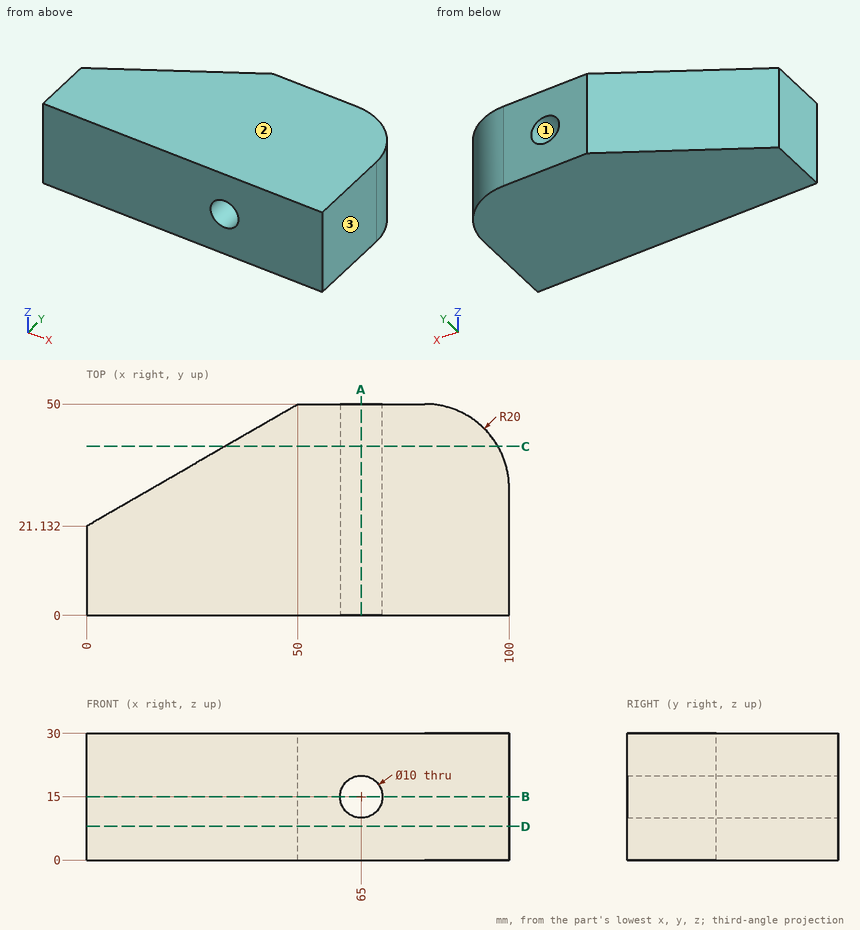
Geometry: see drawing. Coordinates: mm, zero at the bounding-box minimum. Coordinates: 2 decimals unless noted, no trailing zeros. Order: outer loops, then holes, each group sorted by start corner. A loop starts at its lowest first (then second) coordinate and runs counter-clockwise, first axis right, second up. Notation, with made-up numbers: M 67,61.5 L 94,61.5 A14 ccw 94,83.5 Z; hole C 12,51.5 d1. An arc over 180 degrees is marked long. Answer in a Markdown table with one row per item. Add a question column.
Q1. Section query B-B on z = 15. Return the cut outline in (x, y).
Q2. Line query: L1, parallel to Z at x = 65, y = 20; L2, parallel to X at y = 40, z = 16 (1 decimal); L3, parallel to Z at x = 66.5, y = 8. Output: solid intervals per line, ascending.
Q3. Mould query, pull axis Z, two halves, no side actions, for the marked faces 1, 2 and 3. Classes: released by +Z, released by -Z, zero draft, split by the parting line, or undercut.
Q4. Section query D-D on z = 8. Return the cut outline in (x, y), and give its area (3 significant figures).
Q5. Contact query for a flat-ended pin moving along its axis: P1, Ø8, axis at y = 44.5, z = 22, coming from the +X side. Output: stop coordinate, or through.
Q6. Section query C-C on y = 40. Return the cut outline in (x, z).
Q7. Section query A-A on x = 65. Return the cut outline in (y, z), and give its area (3 significant figures).
Completed:
| question | item | result |
|---|---|---|
| 1 | outline | M 0,0 L 60,0 L 60,50 L 50,50 L 0,21.13 Z; M 70,0 L 100,0 L 100,30 A20 ccw 80,50 L 70,50 Z |
| 2 | L1 | z = 0 to 10, 20 to 30 |
| 2 | L2 | x = 32.7 to 60.1, 69.9 to 97.3 |
| 2 | L3 | z = 0 to 10.23, 19.77 to 30 |
| 3 | face 1 | undercut |
| 3 | face 2 | released by +Z |
| 3 | face 3 | zero draft |
| 4 | outline | M 0,0 L 100,0 L 100,30 A20 ccw 80,50 L 50,50 L 0,21.13 Z |
| 4 | area | 4,190 mm2 |
| 5 | P1 | stops at x = 97.02 |
| 6 | outline | M 32.68,0 L 97.32,0 L 97.32,30 L 32.68,30 Z; hole C 65,15 d10 |
| 7 | outline | M 0,0 L 50,0 L 50,10 L 0,10 Z; M 0,20 L 50,20 L 50,30 L 0,30 Z |
| 7 | area | 1,000 mm2 |
